Geometry: final body of the model. Coordinates: model frame, mm. Face numbers are marked on the shaded views. Give positions to 0.01 mm unless a question says otherwise; leave off trailing zeros. Answer as a JSON object with one key per item and string values.
from build123d import *

# Parameters (mm, degrees)
PUNO_PROFILE_R         = 16
COLLARIN_PROFILE_R     = 18
AGUJERO_PUNO_PROFILE_R = 11.1


with BuildPart() as part:
    # Puno: sweep along a curve in space
    with BuildLine() as puno_path:
        Line((250.773980371, 39.928614124, -26.455404118), (379.480094057, 26.797990404, -39.196009311))
    # Puno profile (on start of the path) → Puno (sweep)
    with BuildSketch(Plane(origin=(250.773980371, 39.928614124, -26.455404118), x_dir=(0.10149339146789087, 0.9948362133981381, 0), z_dir=(0.9900470283507966, -0.10100479784184896, -0.09800465533169501))):
        Circle(PUNO_PROFILE_R)
    sweep(path=puno_path.line)

    # Collarin: sweep along a curve in space
    with BuildLine() as collarin_path:
        Line((250.773980371, 39.928614124, -26.455404118), (256.714262541, 39.322585337, -27.04343205))
    # Collarin profile (on start of the path) → Collarin (sweep)
    with BuildSketch(Plane(origin=(250.773980371, 39.928614124, -26.455404118), x_dir=(0.10149339146789053, 0.994836213398138, 0), z_dir=(0.9900470283507966, -0.10100479784184864, -0.09800465533169435))):
        Circle(COLLARIN_PROFILE_R)
    sweep(path=collarin_path.line)

    # Agujero_puno: sweep along a curve in space
    with BuildLine() as agujero_puno_path:
        Line((249.783933343, 40.029618922, -26.357399462), (377.5, 27, -39))
    # Agujero_puno profile (on start of the path) → Agujero_puno (sweep, cut)
    with BuildSketch(Plane(origin=(249.783933343, 40.029618922, -26.357399462), x_dir=(0.10149339146789084, 0.994836213398138, 0), z_dir=(0.9900470283507965, -0.10100479784184893, -0.09800465533169501))):
        Circle(AGUJERO_PUNO_PROFILE_R)
    sweep(path=agujero_puno_path.line, mode=Mode.SUBTRACT)


solid = part.part
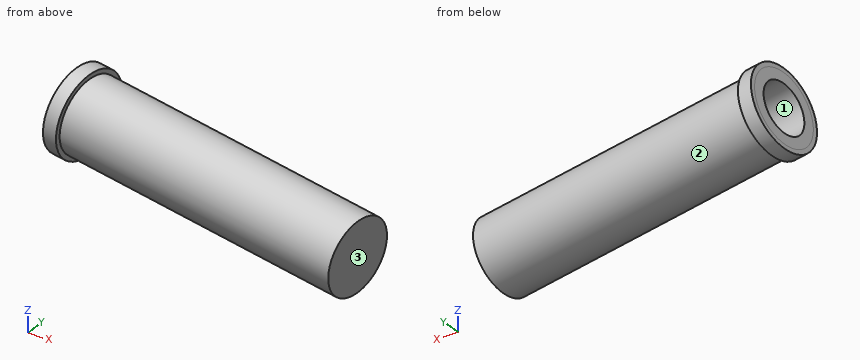
Q1. Material intervals for L1, parallel to Y at x = 255.5, z = -36.5; L2, parallel to Z at x = 294.5, y = 36; L3, parallel to Z at x = 292.5, y = 41, sorted ascending. Write a range as from..to.
Values:
{"L1": "26.43..33.63, 45.07..54.7", "L2": "-46.85..-41.92, -19.64..-14.71", "L3": "-45.7..-40.33, -20.73..-15.36"}
Q2. Mould query, pull axis Z, two halves, no side actions, for the marked faces 1, 2 and 3. Classes: pulls with the +Z half, pulls with the -Z half, needs draft (parallel to the pull), parting line crosses it, or undercut.
Values:
{"face 1": "undercut", "face 2": "parting line crosses it", "face 3": "pulls with the -Z half"}
Q3. First-contact query: P1, Ø4, axis at x = 356, y = 45, coming from the -Z side; P2, Ø12, axis at y = 38.5, z = -23.5, coming from the +X side; P3, Ø3, axis at y = 26, z = -26, coming from the -X side; P4, Ø5, axis at x = 276.5, y = 40.5, coming from the -Z side. Flat tips, straight axial feed; report the tip coordinate or a pass-through.
Values:
{"P1": "z = -44.98", "P2": "x = 381.73", "P3": "x = 249.18", "P4": "z = -45.16"}
